```python
from build123d import *

# Parameters (mm, degrees)
F1_DEPTH = 48
F3_DEPTH = 25


with BuildPart() as f1:
    # F0 (on Top) → F1 (new body)
    with BuildSketch(Plane.XY):
        Polygon((-21.110913, 0), (0, 0), (0, 144.050253), (-4.75, 144.050253), (-9.699747, 149), (-21.464466, 149), (-25, 145.464466), (-25, 3.889087), align=None)
    extrude(amount=F1_DEPTH)

    # F2 (on face) → F3 (cut, through all)
    with BuildSketch(Plane(origin=(-25, 0, 0), x_dir=(0, -1, 0), z_dir=(-1, 0, 0))):
        Polygon((-145.464466, 48), (-145.464466, 24.641155), (-86.190659, 43.772807), (-31.202125, 42.649837), (-3.889087, 26.931672), (-3.889087, 48), align=None)
        Polygon((-116.389087, 7.758158), (-123.464466, 0), (-3.889087, 0), (-3.889087, 7.758158), align=None)
        Polygon((-149, 23.5), (-145.464466, 24.641155), (-145.464466, 48), (-149, 48), align=None)
        Polygon((0, 48), (-3.889087, 48), (-3.889087, 26.931672), (0, 24.693572), align=None)
        Polygon((-3.889087, 7.758158), (-3.889087, 0), (0, 0), (0, 12.693572), (-3.889087, 11.758158), align=None)
    extrude(amount=-F3_DEPTH, mode=Mode.SUBTRACT)

    # F4: F1 across plane


with BuildPart() as f1_1:
    add(f1.part)
    add(f1.part.mirror(Plane.YZ))


solid = f1_1.part
```
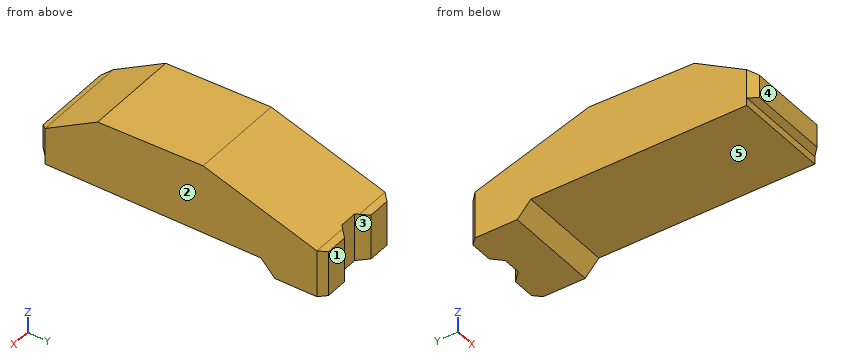
Source: CAD feature listing. Evaluate the final solid. Frame: model axes, mm. Face numbers are marked on the shaded views. A direction names the side the tool comes from. Round coordinates to 2 decimals unless told otherwise and drop trailing zeros. Order: outer loops, then holes, each group sorted by start corner. A loop starts at its lowest first (then second) coordinate and runs counter-clockwise, first axis right, second up. Notation, with made-up numbers: (57, -34) -> (82, -34) arc R22 ccw to (82, -19) -> close; hole circle Ø3 at (13, 81.25). An arc over 180 degrees is marked (long way). One line per item, written item: value. Start each with the question number.
Q1. Section query B-B (z = 6). Return the cut outline in (x, y), plus the area to 3 significant figures.
Q2. Section query A-A (x = 15.5). Return the cut outline in (y, z), plus the area to 3 significant figures.
Q3. Section query C-C (y = 99). Return the cut outline in (x, z), plus the area to 3 significant figures.
Q4. Material intervals for probe 1 along Y at (x, z) = (-0.5, 21); probe 2 along Y at (x, z) = (11, 8); probe 3 along Z at (x, y) = (-6, 15.5), sorted ascending.
Q5. Pin query (flat end, axial travel): pin 1 (1.2 mm diameter, centred on x = 6, z = 10.5, fed in from -Y); pin 2 (1.5 mm diameter, centred on x = -2, y = 18.5, fed in from +Z); pin 3 (10 mm diameter, centred on x = 4, y = 33, fed in from +Z). Return the tip coordinate at first contact, or that it passes through.
Q6. Access query for the marked faces 4 and 5. Directions: +Z, -Z, +X, -X, +Y, -Y. A direction counts if a zero-diameter tool reaches every point of the face in a straight line with its end or side. Return the directions, or none.
Q7. Section query D-D (y = 22.5). Return the cut outline in (x, z), plus the area to 3 significant figures.
Q8. Draft query along X for the marked faces 1, 2 and 3. Return one class per face: pulls with the +X half, pulls with the -X half, needs draft (parallel to the pull), parting line crosses it, or undercut.
Findings below:
1. outline: (-25, 117.99) -> (25, 117.99) -> (25, 145.46) -> (21.46, 149) -> (9.7, 149) -> (4.75, 144.05) -> (-4.75, 144.05) -> (-9.7, 149) -> (-21.46, 149) -> (-25, 145.46) -> close
1. area: 1,470 mm²
2. outline: (0, 12.69) -> (3.89, 11.76) -> (3.89, 7.76) -> (116.39, 7.76) -> (123.46, 0) -> (149, 0) -> (149, 23.5) -> (86.19, 43.77) -> (31.2, 42.65) -> (0, 24.69) -> close
2. area: 4,590 mm²
3. outline: (-25, 7.76) -> (25, 7.76) -> (25, 39.64) -> (-25, 39.64) -> close
3. area: 1,590 mm²
4. probe 1: 0 to 144.05
4. probe 2: 3.89 to 149
4. probe 3: 7.76 to 33.61
5. pin 1: y = 3.89
5. pin 2: z = 35.77
5. pin 3: z = 42.79
6. face 4: +Z, -Z, +X, -X, -Y
6. face 5: -Z, +X, -X, -Y
7. outline: (-25, 7.76) -> (25, 7.76) -> (25, 37.64) -> (-25, 37.64) -> close
7. area: 1,490 mm²
8. face 1: needs draft
8. face 2: pulls with the +X half
8. face 3: undercut
